Job drawing, mm, ordinate dimensions from the low corner. One solid piece. Round coordinates to 2 decimals unless told otherwise and drop trailing zeros. Loops run counter-clockwise (first coordinate to the right, second up) from the corner with the lowest first, then second, coordinate; pieces in that order, holes last.
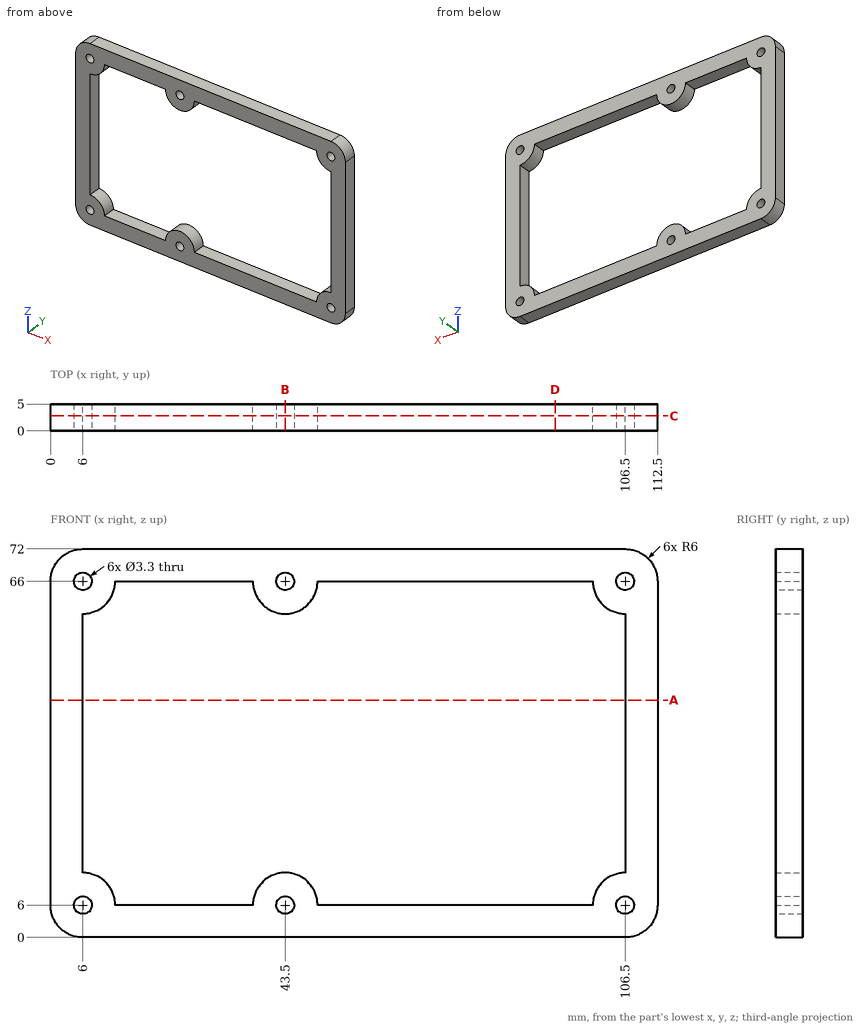
Item 1: Flat gauge pin, fed straight in: P1, Ø4.5, axis at x = 43.5, z = 66, coming from the -Y side. Where does the tip first touch, or does it go through?
Answers follow:
P1: stops at y = 0
Item 2: Cut at D-D, the plane x = 93.5. Give the cut face in (y, z).
Answers follow:
outline: (0, 0) - (5, 0) - (5, 6) - (0, 6) - close; (0, 66) - (5, 66) - (5, 72) - (0, 72) - close
Item 3: Cut at A-A, the plane z = 44. Give the cut face in (x, y).
Answers follow:
outline: (0, 0) - (6, 0) - (6, 5) - (0, 5) - close; (106.5, 0) - (112.5, 0) - (112.5, 5) - (106.5, 5) - close
Item 4: Cut at C-C, the plane y = 2.8. Give the cut face in (x, z), plus the area to 3 significant figures.
Answers follow:
outline: (0, 6) arc R6 ccw to (6, 0) - (106.5, 0) arc R6 ccw to (112.5, 6) - (112.5, 66) arc R6 ccw to (106.5, 72) - (6, 72) arc R6 ccw to (0, 66) - close; hole circle Ø3.3 at (6, 6); hole circle Ø3.3 at (6, 66); hole (6, 12) arc R6 cw to (12, 6) - (37.5, 6) arc R6 cw to (49.5, 6) - (100.5, 6) arc R6 cw to (106.5, 12) - (106.5, 60) arc R6 cw to (100.5, 66) - (49.5, 66) arc R6 cw to (37.5, 66) - (12, 66) arc R6 cw to (6, 60) - close; hole circle Ø3.3 at (43.5, 6); hole circle Ø3.3 at (43.5, 66); hole circle Ø3.3 at (106.5, 6); hole circle Ø3.3 at (106.5, 66)
area: 2,210 mm2
Item 5: Cut at B-B, the plane x = 43.5. Give the cut face in (y, z), plus the area to 3 significant figures.
Answers follow:
outline: (0, 0) - (5, 0) - (5, 4.35) - (0, 4.35) - close; (0, 7.65) - (5, 7.65) - (5, 12) - (0, 12) - close; (0, 60) - (5, 60) - (5, 64.35) - (0, 64.35) - close; (0, 67.65) - (5, 67.65) - (5, 72) - (0, 72) - close
area: 87.0 mm2
Item 6: Probe line 1 (X direction, y = 1, z = 18.5); line 2 (X direction, y = 2.2, z = 62.5); line 3 (Z direction, x = 86, y = 2.3). List the from-to ranges inside material, lowest first.
Answers follow:
line 1: x = 0 to 6, 106.5 to 112.5
line 2: x = 0 to 10.87, 38.63 to 48.37, 101.63 to 112.5
line 3: z = 0 to 6, 66 to 72
